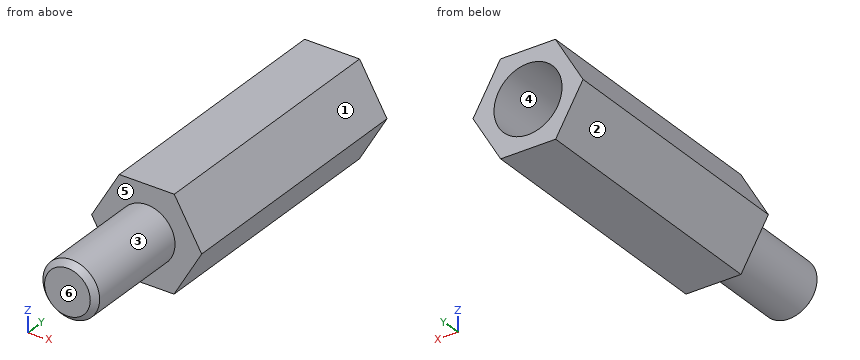
```python
from build123d import *

# Parameters (mm, degrees)
EXTRUDE_1_DEPTH     = 11.7
SKETCH_2_R          = 1.5
CUT_EXTRUDE_1_DEPTH = 10
SKETCH_3_R          = 1.5
EXTRUDE_2_DEPTH     = 5


# Read off the part's stored shape, not the designer's step: M2.5 机械螺纹 螺柱1
with BuildPart() as part:
    # 草图1 → 凸台-拉伸1 (new body)
    with BuildSketch(Plane(origin=(0, 0, 0), x_dir=(1, 0, 0), z_dir=(0, 1, 0))):
        Polygon((-1.21761392, 2.097001751), (-2.424863748, -0.005983711), (-1.207249828, -2.102985462), (1.21761392, -2.097001751), (2.424863748, 0.005983711), (1.207249828, 2.102985462), align=None)
    extrude(amount=EXTRUDE_1_DEPTH)

    # 草图2 → 切除-拉伸1 (cut)
    with BuildSketch(Plane(origin=(0, 11.7, 0), x_dir=(1, 0, 0), z_dir=(0, 1, 0))):
        with Locations(Location((0, 0, 0), (0, 0, 270))):
            Circle(SKETCH_2_R)
    extrude(amount=-CUT_EXTRUDE_1_DEPTH, mode=Mode.SUBTRACT)

    # 草图3 → 凸台-拉伸2 (add)
    with BuildSketch(Plane.XZ):
        with Locations(Location((0, 0, 0), (0, 0, 90))):
            Circle(SKETCH_3_R)
    extrude(amount=EXTRUDE_2_DEPTH)

    # M2.5 机械螺纹 螺柱1 outline → M2.5 机械螺纹 螺柱1 (revolve, cut)
    with BuildSketch(Plane.XY):
        Polygon((1.5, 0), (1.25, 0), (1.25, -4.7565), (1.0065, -5), (1.5, -5), align=None)
    revolve(axis=Axis((0, 0, 0), (0, 1, 0)), mode=Mode.SUBTRACT)


solid = part.part
```
Check sheet for the modelled part. Datum: model origin and axes. Units: mm. Face numbers are marked on the shaded views. A direction names the side the tool comes from. Round coordinates to 2 decimals unless told otherwise and drop trailing zeros. Order: outer loops, then holes, each group sorted by start corner. A loop starts at its lowest first (then second) coordinate and runs counter-clockwise, first axis right, second up.
1) Tool access check on the marked faces 5 and 6. Record the directions out of +Z, -Z, +X, -X, +Y, -Y that give a thin tool (end or side, any length) a straight path to the whole face; none if there is none.
2) Scan lines: line 1 (Y direction, x = 0.25, z = -1.55); line 2 (Y direction, x = -1.45, z = 0.15); line 3 (X direction, y = 3.75, z = -0.9). Record each from-to range of solid material in increasing order.
3) Mould release check, pull along Z, two halves, no side actions. Record for the marked faces 1, 2, 3 and 4: +Z half, -Z half, draft (parallel to the pull), parting line (faces both ways), or undercut.
4) Section check B-B (x = 0). Record the boundary of the cut face in (y, z), and give its area (3 significant figures).
5) Section check D-D (x = -1.95). Record the boundary of the cut face in (y, z).
6) Section check A-A (y = 9). Record the boundary of the cut face in (x, z), and give its area (3 significant figures).
7) Section check C-C (y = -3.5). Record the boundary of the cut face in (x, z).
8) Go/stop test with flat-tipped pins: pin 1 Ø2 at (y, z) = (-2.5, 1.5) entering from +X; pin 2 Ø1.5 at (x, y) = (1, 3.5) entering from +Z. Record where each tip stops, or that it passes through.
Result:
1. face 5: -Y
1. face 6: +Z, -Z, +X, -X, -Y
2. line 1: y = 0 to 11.7
2. line 2: y = 0 to 1.7
2. line 3: x = -1.9 to -1.2, 1.2 to 1.91
3. face 1: +Z half
3. face 2: -Z half
3. face 3: parting line
3. face 4: undercut
4. outline: (-5, -1.01) - (-4.76, -1.25) - (0, -1.25) - (0, -2.1) - (11.7, -2.1) - (11.7, -1.5) - (1.7, -1.5) - (1.7, 1.5) - (11.7, 1.5) - (11.7, 2.1) - (0, 2.1) - (0, 1.25) - (-4.76, 1.25) - (-5, 1.01) - close
4. area: 31.6 mm2
5. outline: (0, -0.82) - (11.7, -0.82) - (11.7, 0.82) - (0, 0.82) - close
6. outline: (-2.42, 0.01) - (-1.22, -2.1) - (1.21, -2.1) - (2.42, -0.01) - (1.22, 2.1) - (-1.21, 2.1) - close; hole circle Ø3 at (0, 0)
6. area: 8.21 mm2
7. outline: circle Ø2.5 at (0, 0)
8. pin 1: stops at x = 1.15
8. pin 2: stops at z = 2.1
